Design review of the part built by this model. Coordinates are the model's own, in mm. A direction names the side the tool comes from. Give positions to 0.01 mm unless a question says otherwise; leave off trailing zeros. Write each loop counter-clockwise with the first axis right and the second up, starting at its lowest first coordinate (ties: lowest second). Pieces come first, ordered by that corner, then holes. Notation, with made-up numbers: M 32,-1 L 58,-1 A24 ccw 58,27 Z; hole C -18,-1 d6. An arc over 180 degrees is marked long. Answer in a Markdown table with one row per item.
```python
from build123d import *

# Parameters (mm, degrees)
ESQUISSE2_R             = 6.75
ENL_V_MAT_EXTRU_1_DEPTH = 340.011061766


with BuildPart() as part:
    # Esquisse1 → Révolution1 (revolve)
    with BuildSketch(Plane.XY, mode=Mode.PRIVATE) as r_volution1_sk:
        with BuildLine():
            Line((-237.5, 0), (-237.5, 46))
            Line((-237.5, 46), (-200.5, 46))
            Line((-200.5, 46), (-200.5, 40))
            Line((-200.5, 40), (-203.5, 40))
            Line((-203.5, 40), (-203.5, 37))
            Line((-203.5, 37), (-200.5, 37))
            Line((-200.5, 37), (-200.5, 30))
            ThreePointArc((-200.5, 30), (-206.833651811, 27.738530528), (-210.302631579, 21.976970948))
            ThreePointArc((-210.302631579, 21.976970948), (-212, 20), (-210.302631579, 18.023029052))
            ThreePointArc((-210.302631579, 18.023029052), (-206.833651811, 12.261469472), (-200.5, 10))
            Line((-200.5, 10), (-200.5, 0))
            Line((-200.5, 0), (-237.5, 0))
        make_face()
    revolve(r_volution1_sk.sketch.rotate(Axis((0, 46, 0), (0, -1, 0)), 270), axis=Axis((0, 46, 0), (0, -1, 0)))

    # Esquisse2 → Enlèv. mat.-Extru.1 (cut, through all)
    with BuildSketch(Plane(origin=(0, 46, 0), x_dir=(1, 0, 0), z_dir=(0, 1, 0))):
        with Locations(Location((-224, 0, 0), (0, 0, 270))):
            Circle(ESQUISSE2_R)
        with Locations(Location((-206.949015283, 85.72108885, 0), (0, 0, 270))):
            Circle(ESQUISSE2_R)
        with Locations(Location((-158.391918986, 158.391918986, 0), (0, 0, 270))):
            Circle(ESQUISSE2_R)
        with Locations(Location((-85.72108885, 206.949015283, 0), (0, 0, 270))):
            Circle(ESQUISSE2_R)
        with Locations(Location((0, 224, 0), (0, 0, 270))):
            Circle(ESQUISSE2_R)
        with Locations(Location((85.72108885, 206.949015283, 0), (0, 0, 270))):
            Circle(ESQUISSE2_R)
        with Locations(Location((158.391918986, 158.391918986, 0), (0, 0, 270))):
            Circle(ESQUISSE2_R)
        with Locations(Location((206.949015283, 85.72108885, 0), (0, 0, 270))):
            Circle(ESQUISSE2_R)
        with Locations(Location((224, 0, 0), (0, 0, 270))):
            Circle(ESQUISSE2_R)
        with Locations(Location((206.949015283, -85.72108885, 0), (0, 0, 270))):
            Circle(ESQUISSE2_R)
        with Locations(Location((158.391918986, -158.391918986, 0), (0, 0, 270))):
            Circle(ESQUISSE2_R)
        with Locations(Location((85.72108885, -206.949015283, 0), (0, 0, 270))):
            Circle(ESQUISSE2_R)
        with Locations(Location((0, -224, 0), (0, 0, 270))):
            Circle(ESQUISSE2_R)
        with Locations(Location((-85.72108885, -206.949015283, 0), (0, 0, 270))):
            Circle(ESQUISSE2_R)
        with Locations(Location((-158.391918986, -158.391918986, 0), (0, 0, 270))):
            Circle(ESQUISSE2_R)
        with Locations(Location((-206.949015283, -85.72108885, 0), (0, 0, 270))):
            Circle(ESQUISSE2_R)
    extrude(amount=-ENL_V_MAT_EXTRU_1_DEPTH, mode=Mode.SUBTRACT)


solid = part.part
```
1) Insertion check: P1, Ø1.5, axis at y = 20.5, z = 124, coming from the -X side; P2, Ø3, axis at y = 17, z = -111.5, coming from the +X side; P3, Ø10, axis at x = -155, y = 27, coming from the -Z side. Each pin has a flat end and moves straight along its axis. Give the tip position at first contact, or say it passes through.
Geometry says:
| item | result |
|---|---|
| P1 | x = -203.02 |
| P2 | x = 210.49 |
| P3 | z = -184.14 |
2) The part is to be moulded in two halves that separate along Z. For faces 3 (the face through (-2.585, 23.322, -217.765)), 4 (the face through (-142, 0, 142)), 5 (the face through (-71.339, 23.322, 226.533)), say which applies: released by +Z, released by -Z, zero draft, split by the parting line, or undercut.
Geometry says:
| item | result |
|---|---|
| face 3 | undercut |
| face 4 | zero draft |
| face 5 | split by the parting line |
3) To check wall thickness, follow probe 1 along Z at (x, y) = (208, 32); probe 2 along Y at (x, z) = (128.5, -157); probe 3 along X at (y, z) = (11.5, -87.5). State the ranges of each line that lie inside material, in increasing order. Write a range as [from, to].
Geometry says:
| item | result |
|---|---|
| probe 1 | [-114.64, -92.39], [-79.05, 79.05], [92.39, 114.64] |
| probe 2 | [0, 10.29], [29.71, 37], [40, 46] |
| probe 3 | [-220.79, -213.46], [-200.44, -186.24], [186.24, 200.44], [213.46, 220.79] |
4) Add section C-C (x = 224). Write out the cut boundary in (y, z), and give its area (3 significant figures).
Geometry says:
| item | result |
|---|---|
| outline | M 0,-78.93 L 46,-78.93 L 46,-6.75 L 0,-6.75 Z; M 0,6.75 L 46,6.75 L 46,78.93 L 0,78.93 Z |
| area | 6,640 mm^2 |
5) Add section A-A (z = 0). Count the separate pieces of the cut face and the enclosed holes in it, and give its area (3 significant figures).
Geometry says:
| item | result |
|---|---|
| separate pieces | 4 |
| enclosed holes | 0 |
| area | 1,820 mm^2 |
6) Add section D-D (z = 224). Write out the cut boundary in (x, y), and give its area (3 significant figures).
Geometry says:
| item | result |
|---|---|
| outline | M -78.93,0 L -6.75,0 L -6.75,46 L -78.93,46 Z; M 6.75,0 L 78.93,0 L 78.93,46 L 6.75,46 Z |
| area | 6,640 mm^2 |
7) For faces 1 (the face through (-85.424, 23.322, -213.692)), 2 (the face through (198.66, 38.48, -44.11)), list the 3-axis set-ups (+Z, -Z, +X, -X, +Y, -Y) from which the entire face can be reached by the end or side of a thin tool; tool diameter is ignored.
Geometry says:
| item | result |
|---|---|
| face 1 | +Y, -Y |
| face 2 | none |
